Part model, mm, in its own coordinate system. Face numbers are marked on the shaded views. Round coordinates to 2 decimals unless told otherwise and drop trailing zeros. Write each loop counter-clockwise with the first axis right and the second up, starting at its lowest first coordinate (ties: lowest second). Pieces come first, ordered by that corner, then holes. Notation, with made-up numbers: (-17.5, 53.25) -> (33.5, 53.25) arc R10 cw to (33.5, 58.25) -> close; hole circle Ø8 at (47, 24). An arc over 180 degrees is marked (long way). Return JSON: item names as keys, results as strings. Group by question number.
Autodesk Inventor part; units mm, degrees
ref_plane "YZ Plane" through (0, 0, 0) normal (1, 0, 0) x (0, 1, 0)
ref_plane "XZ Plane" through (0, 0, 0) normal (0, 1, 0) x (-1, 0, 0)
ref_plane "XY Plane" through (0, 0, 0) normal (0, 0, 1) x (1, 0, 0)
sketch "Sketch1" plane through (0, 0, 0) normal (0, 1, 0) x (-1, 0, 0)
  circle A0 centre (1.143, 0) radius 39 construction
  circle A1 centre (1.143, 0) radius 42
  line L0 (-21.857, 14) -> (-36.857, 14) construction
  line L1 (-36.857, 14) -> (-36.857, 5) construction
  line L2 (-36.857, 5) -> (-21.857, 5) construction
  line L3 (-21.857, 5) -> (-21.857, 14) construction
  line L4 (1.143, 0) -> (-37.857, 0)
  line L5 (0, 0) -> (0, -22) construction
  dimension "d0" = 78
  dimension "d1" = 9
  dimension "d2" = 15
  dimension "d3" = 5
  dimension "d4" = 23
  dimension "d5" = 84
  dimension "d11" = 1.143
extrude "Extrusion1" add sketch "Sketch1" along normal blind 6
fillet "Fillet1" radius 7 1 edges at (40.857, 0, 0)
shell "Shell1" thickness 2 removed faces 1 at (-4.0377, 6, 12.235)
sketch "Sketch2" plane through (-1.143, 2, 0) normal (0, 1, 0) x (1, 0, 0)
  circle A0 centre (-11.303, -22.606) radius 1.95
  circle A1 centre (18.034, 6.223) radius 1.95
  circle A2 centre (-11.303, -22.606) radius 3.5
  circle A3 centre (18.034, 6.223) radius 3.5
  point P0 (1.143, 0)
  dimension "d12" = 3.9
  dimension "d13" = 3.9
  dimension "d14" = 6.223
  dimension "d15" = 16.891
  dimension "d16" = 22.606
  dimension "d17" = 12.446
  dimension "d18" = 7
  dimension "d19" = 7
extrude "Extrusion2" add sketch "Sketch2" along normal blind 5.5
sketch "Sketch3" plane through (-1.143, 2, 0) normal (0, 1, 0) x (1, 0, 0)
  line L0 (7.5, 19.5) -> (-25.5, 19.5) construction
  line L1 (-25.5, 19.5) -> (-25.5, -9.5) construction
  line L2 (-25.5, -9.5) -> (7.5, -9.5) construction
  line L3 (7.5, -9.5) -> (7.5, 19.5) construction
  line L4 (7.5, 19.5) -> (-25.5, -9.5) construction
  line L5 (-25.5, 19.5) -> (7.5, -9.5) construction
  point P0 (1.143, 0)
  point P1 (-9, 5)
  dimension "d22" = 33
  dimension "d23" = 29
sketch "Sketch5" plane through (-1.143, 6, 0) normal (0, 1, 0) x (1, 0, 0)
  line L0 (31.143, -15) -> (45, -15)
  line L1 (45, -15) -> (45, -3)
  line L2 (45, -3) -> (31.143, -3)
  line L3 (31.143, -3) -> (31.143, -15)
  line L4 (1.143, 0) -> (-32, 0) construction
  line L5 (31.143, 15) -> (45, 15)
  line L6 (45, 15) -> (45, 3)
  line L7 (45, 3) -> (31.143, 3)
  line L8 (31.143, 3) -> (31.143, 15)
  dimension "d24" = 3
  dimension "d25" = 12
  dimension "d26" = 30
extrude "Extrusion3" cut sketch "Sketch5" against normal up to surface (4 mm away)
properties part number "Case bottom"
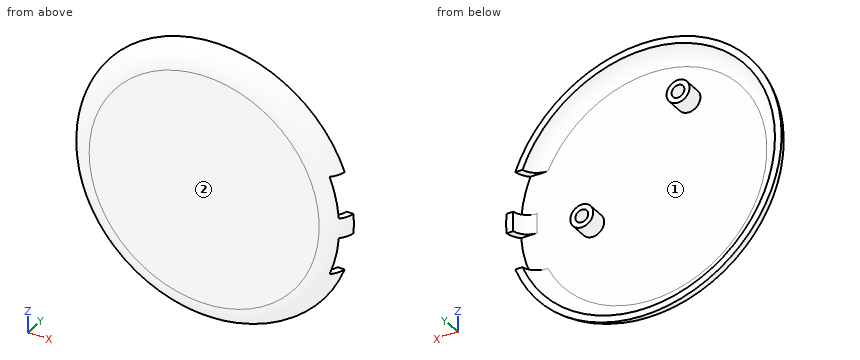
Item 1: Flat gauge pins, fed straight in: P1, Ø2, axis at x = 34.5, y = 4, coming from the -Z side; P2, Ø1.2, axis at x = -13, z = 22, coming from the +Y side; P3, Ø2, axis at x = 36.5, y = 3, coming from the +Z side. Where does each tip first touch, or does it go through?
Item 2: Cut at A-A (y = 4). Write the cut outline in (x, z).
Item 3: Wall check: L1, parallel to Z at x = -11.5, y = 3.75; L2, parallel to Y at x = -29, z = 15; L3, parallel to Z at x = -14.5, y = 3.5. Give the ranges that are in metal, low to high.
Item 4: Two-plate mould, pull along Z, no slides. Class the marked faces 1 and 2: released by +Z, released by -Z, zero draft, split by the parting line, or undercut.
Checks:
{
 "1": {"P1": "stops at z = -22.85", "P2": "stops at y = 2", "P3": "stops at z = 18.43"},
 "2": {"outline": "circle Ø7 at (-12.45, 22.61); circle Ø7 at (16.89, -6.22); (34.93, -15) arc R39.07 cw (long way) to (34.93, 15) -> (37.44, 15) arc R41.4 ccw (long way) to (37.44, -15) -> close; (37.81, -3) -> (40.14, -3) arc R41.4 ccw to (40.14, 3) -> (37.81, 3) arc R39.07 cw to start; hole circle Ø3.9 at (-12.45, 22.61); hole circle Ø3.9 at (16.89, -6.22)"},
 "3": {"L1": "z = -39.95 to -37.47, 19.24 to 20.9, 24.31 to 25.98, 37.47 to 39.95", "L2": "y = 0 to 2", "L3": "z = -38.9 to -36.26, 19.77 to 25.44, 36.26 to 38.9"},
 "4": {"face 1": "undercut", "face 2": "zero draft"}
}
